```python
from build123d import *

# Parameters (mm, degrees)
SQUARE_TUBE_20_X_20_X_2_1_DEPTH                     = 110
SKETCH2_W                                           = 40
SKETCH2_H                                           = 30
BOSS_EXTRUDE1_DEPTH                                 = 5
CSK_FOR_M3_COUNTERSUNK_FLAT_HEAD_SCREW1_D           = 3.4
CSK_FOR_M3_COUNTERSUNK_FLAT_HEAD_SCREW1_DEPTH       = 30
CSK_FOR_M3_COUNTERSUNK_FLAT_HEAD_SCREW1_CSINK_D     = 6.3
CSK_FOR_M3_COUNTERSUNK_FLAT_HEAD_SCREW1_CSINK_ANGLE = 90
CSK_FOR_M3_COUNTERSUNK_FLAT_HEAD_SCREW1_TIP         = 1.021463052
SKETCH5_R                                           = 0.9
CUT_EXTRUDE1_DEPTH                                  = 5
CUT_EXTRUDE2_START                                  = -5
SKETCH6_R                                           = 0.9
CUT_EXTRUDE2_DEPTH                                  = 5


with BuildPart() as part:
    # Sketch1 → Square tube 20 X 20 X 2(1) (new body)
    with BuildSketch(Plane(origin=(0, 0, 0), x_dir=(1, 0, 0), z_dir=(0, 1, 0))):
        with BuildLine():
            Line((-6, -10), (6, -10))
            ThreePointArc((6, -10), (8.828427125, -8.828427125), (10, -6))
            Line((10, -6), (10, 6))
            ThreePointArc((10, 6), (8.828427125, 8.828427125), (6, 10))
            Line((6, 10), (-6, 10))
            ThreePointArc((-6, 10), (-8.828427125, 8.828427125), (-10, 6))
            Line((-10, 6), (-10, -6))
            ThreePointArc((-10, -6), (-8.828427125, -8.828427125), (-6, -10))
        make_face()
        with BuildLine():
            Line((-6, -8), (6, -8))
            ThreePointArc((6, -8), (7.414213562, -7.414213562), (8, -6))
            Line((8, -6), (8, 6))
            ThreePointArc((8, 6), (7.414213562, 7.414213562), (6, 8))
            Line((6, 8), (-6, 8))
            ThreePointArc((-6, 8), (-7.414213562, 7.414213562), (-8, 6))
            Line((-8, 6), (-8, -6))
            ThreePointArc((-8, -6), (-7.414213562, -7.414213562), (-6, -8))
        make_face(mode=Mode.SUBTRACT)
    extrude(amount=SQUARE_TUBE_20_X_20_X_2_1_DEPTH)

    # Sketch2 → Boss-Extrude1 (add)
    with BuildSketch(Plane(origin=(0, 0, 0), x_dir=(1, 0, 0), z_dir=(0, 1, 0))):
        Rectangle(SKETCH2_W, SKETCH2_H)
    extrude(amount=-BOSS_EXTRUDE1_DEPTH)

    # CSK for M3 Countersunk Flat Head Screw1
    with Locations(Plane(origin=(0, 0, 0), x_dir=(1, 0, 0), z_dir=(0, 1, 0))):
        with Locations((15, 10), (-15, 10), (-15, -10), (15, -10)):
            CounterSinkHole(CSK_FOR_M3_COUNTERSUNK_FLAT_HEAD_SCREW1_D / 2, CSK_FOR_M3_COUNTERSUNK_FLAT_HEAD_SCREW1_CSINK_D / 2, depth=CSK_FOR_M3_COUNTERSUNK_FLAT_HEAD_SCREW1_DEPTH, counter_sink_angle=CSK_FOR_M3_COUNTERSUNK_FLAT_HEAD_SCREW1_CSINK_ANGLE)
            with Locations((0, 0, -(CSK_FOR_M3_COUNTERSUNK_FLAT_HEAD_SCREW1_DEPTH + CSK_FOR_M3_COUNTERSUNK_FLAT_HEAD_SCREW1_TIP / 2))):  # 118° drill point
                Cone(0, CSK_FOR_M3_COUNTERSUNK_FLAT_HEAD_SCREW1_D / 2, CSK_FOR_M3_COUNTERSUNK_FLAT_HEAD_SCREW1_TIP, mode=Mode.SUBTRACT)

    # Sketch5 → Cut-Extrude1 (cut)
    with BuildSketch(Plane(origin=(0, 0, -10), x_dir=(-1, 0, 0), z_dir=(0, 0, -1))):
        with Locations((2.999999983, 66.1)):
            Circle(SKETCH5_R)
        with Locations((2.999999983, 58.1)):
            Circle(SKETCH5_R)
        with Locations((-7.000000017, 58.1)):
            Circle(SKETCH5_R)
        with Locations((-7.000000017, 66.1)):
            Circle(SKETCH5_R)
    extrude(amount=-CUT_EXTRUDE1_DEPTH, mode=Mode.SUBTRACT)

    # Sketch6 → Cut-Extrude2 (cut)
    with BuildSketch(Plane.XY.offset(10).offset(CUT_EXTRUDE2_START)):
        with Locations(Location((-2.999999994, 66.1, 0), (0, 0, 180))):
            Circle(SKETCH6_R)
        with Locations(Location((7.000000006, 66.1, 0), (0, 0, 180))):
            Circle(SKETCH6_R)
        with Locations(Location((7.000000006, 58.1, 0), (0, 0, 180))):
            Circle(SKETCH6_R)
        with Locations(Location((-2.999999994, 58.1, 0), (0, 0, 180))):
            Circle(SKETCH6_R)
    extrude(amount=CUT_EXTRUDE2_DEPTH, mode=Mode.SUBTRACT)


solid = part.part
```
For this review, take the finished solid that the model builds, in its own axes (mm). A direction names the side the tool comes from. Coordinates: 2 decimals unless noted, no trailing zeros. Order: outer loops, then holes, each group sorted by start corner. A loop starts at its lowest first (then second) coordinate and runs counter-clockwise, first axis right, second up. Notation, with made-up numbers: (36.25, 55) -> (82.25, 55) arc R18 cw to (82.25, 78) -> close; hole circle Ø5 at (28.5, 39.5). An arc over 180 degrees is marked (long way). Use CSV: the item, a comma, the result in double quotes. Start each with the question number.
Item 1: We need section B-B, the plane y = 88.5. Give the boundary of the cut face in (x, z).
Item 2: For faces 1 (the face through (0, 54, -10)), 2 (the face through (0, 54, -8)), 3 (the face through (-10, 54, 0)), list the 3-axis set-ups (+Z, -Z, +X, -X, +Y, -Y) from which the entire face can be reached by the end or side of a thin tool; tool diameter is ignored.
Item 3: Wall thickness on probe 1 along Y at (x, z) = (-3, 8.55); probe 2 along Z at (x, y) = (-15, -3.8); probe 3 along X at (y, z) = (-3.6, 10): over which ranges is each line inside the solid? List them lowest first.
Item 4: Insertion check: pin 1 (6 mm diameter, centred on x = -1, y = 28.5, fed in from -Z); pin 2 (1 mm diameter, centred on y = 97.5, z = 5, fed in from -X); pin 3 (3 mm diameter, centred on x = -15, z = 10, fed in from -Y); pin 4 (4 mm diameter, centred on y = 89, z = -9.5, fed in from -X). Each pin has a flat end and moves straight along its axis. Give the tip position at first contact, or say it passes through.
Item 5: We need section C-C, the plane z = 4. Give the boundary of the cut face in (x, y), then the cut area to 3 significant figures.
Item 6: Draft analysis for pull direction Z (two halves, no side actions). For faces 4 (the face through (-8.859, 54.23, 8.797)), 5 (the face through (7.43, 54.23, -7.4)), 6 (the face through (0, -2, -15)), 7 (the face through (20, -2, 0)), state which applies: pulls with the +Z half, pulls with the -Z half, needs draft (parallel to the pull), parting line crosses it, or undercut.
Item 7: We need section A-A, the plane x = 15. Give the boundary of the cut face in (y, z), then the cut area to 3 significant figures.
Derived:
1,outline,"(-10, -6) arc R4 ccw to (-6, -10) -> (6, -10) arc R4 ccw to (10, -6) -> (10, 6) arc R4 ccw to (6, 10) -> (-6, 10) arc R4 ccw to (-10, 6) -> close; hole (-8, -6) arc R2 ccw to (-6, -8) -> (6, -8) arc R2 ccw to (8, -6) -> (8, 6) arc R2 ccw to (6, 8) -> (-6, 8) arc R2 ccw to (-8, 6) -> close"
2,face 1,"-Z, +X, -X, +Y"
2,face 2,"+Y"
2,face 3,"+Z, -Z, -X, +Y"
3,probe 1,"y = -5 to 57.2, 59 to 65.2, 67 to 110"
3,probe 2,"z = -15 to -11.7, -8.3 to 8.3, 11.7 to 15"
3,probe 3,"x = -20 to -16.7, -13.3 to 13.3, 16.7 to 20"
4,pin 1,"stops at z = -10"
4,pin 2,"stops at x = -10"
4,pin 3,"passes through"
4,pin 4,"stops at x = -9.71"
5,outline,"(-20, -5) -> (20, -5) -> (20, 0) -> (10, 0) -> (10, 110) -> (8, 110) -> (8, 0) -> (-8, 0) -> (-8, 110) -> (-10, 110) -> (-10, 0) -> (-20, 0) -> close"
5,area,"640 mm^2"
6,face 4,"pulls with the +Z half"
6,face 5,"undercut"
6,face 6,"pulls with the -Z half"
6,face 7,"needs draft"
7,outline,"(-5, -15) -> (0, -15) -> (0, -13.15) -> (-1.45, -11.7) -> (-5, -11.7) -> close; (-5, -8.3) -> (-1.45, -8.3) -> (0, -6.85) -> (0, 6.85) -> (-1.45, 8.3) -> (-5, 8.3) -> close; (-5, 11.7) -> (-1.45, 11.7) -> (0, 13.15) -> (0, 15) -> (-5, 15) -> close"
7,area,"112 mm^2"
